```python
from build123d import *
from OCP.BRepFilletAPI import BRepFilletAPI_MakeChamfer

# Parameters (mm, degrees)
SKETCH_1_W          = 23
SKETCH_1_H          = 40
SKETCH_1_R          = 9.5
EXTRUDE_1_DEPTH     = 1.5
FILLET_1_R          = 2
SKETCH_3_R          = 1.15
CUT_EXTRUDE_1_DEPTH = 24.119256043
SKETCH_4_R          = 0.65
EXTRUDE_2_DEPTH     = 2
CHAMFER_1_SIZE      = 2
CHAMFER_1_SIZE_2    = 0.1


with BuildPart() as part:
    # 草图1 → 凸台-拉伸1 (new body)
    with BuildSketch(Plane.XY):
        Rectangle(SKETCH_1_W, SKETCH_1_H)
        with Locations((0, -4.5)):
            Circle(SKETCH_1_R, mode=Mode.SUBTRACT)
    extrude(amount=EXTRUDE_1_DEPTH)

    # 圆角1
    fillet_1_edges = [part.edges().sort_by_distance(p)[0] for p in [
        (11.5, -20, 0.75),
        (-11.5, -20, 0.75),
        (-11.5, 20, 0.75),
        (11.5, 20, 0.75),
    ]]
    fillet(fillet_1_edges, radius=FILLET_1_R)

    # 草图3 → 切除-拉伸1 (cut, through all)
    with BuildSketch(Plane.XY.offset(1.5)):
        with Locations((-8, 18)):
            Circle(SKETCH_3_R)
        with Locations((8, 18)):
            Circle(SKETCH_3_R)
        with Locations((-9, -17)):
            Circle(SKETCH_3_R)
        with Locations((9, -17)):
            Circle(SKETCH_3_R)
    extrude(amount=-CUT_EXTRUDE_1_DEPTH, mode=Mode.SUBTRACT)

    # 草图4 → 凸台-拉伸2 (add)
    with BuildSketch(Plane.XY.offset(1.5)):
        with Locations(Location((-8, -12, 0), (0, 0, 180))):
            Circle(SKETCH_4_R)
        with Locations(Location((8, -12, 0), (0, 0, 180))):
            Circle(SKETCH_4_R)
    extrude(amount=EXTRUDE_2_DEPTH)

    # 倒角1
    chamfer_1_edges_1 = [part.edges().sort_by_distance(p)[0] for p in [
        (-7.35, -12, 3.5),
    ]]
    chamfer_1_side_1 = [part.faces().sort_by_distance(p)[0] for p in [
        (-7.35, -12, 3.498),
    ]]
    chamfer_1_edges_2 = [part.edges().sort_by_distance(p)[0] for p in [
        (8.65, -12, 3.5),
    ]]
    chamfer_1_side_2 = [part.faces().sort_by_distance(p)[0] for p in [
        (8.65, -12, 3.498),
    ]]
    chamfer_1 = BRepFilletAPI_MakeChamfer(part.part.solid().wrapped)
    for e in chamfer_1_edges_1:
        chamfer_1.Add(CHAMFER_1_SIZE - 0.0001, CHAMFER_1_SIZE_2 - 0.0001, e.wrapped, chamfer_1_side_1[0].wrapped)
    for e in chamfer_1_edges_2:
        chamfer_1.Add(CHAMFER_1_SIZE - 0.0001, CHAMFER_1_SIZE_2 - 0.0001, e.wrapped, chamfer_1_side_2[0].wrapped)
    add(Compound.cast(chamfer_1.Shape()), mode=Mode.REPLACE)  # a hair under: the kernel refuses the full size


solid = part.part
```
For this review, take the finished solid that the model builds, in its own axes (mm). Round coordinates to 2 decimals unless told otherwise and drop trailing zeros. Write each loop counter-clockwise with the first axis right and the second up, starting at its lowest first coordinate (ties: lowest second). Pieces come first, ordered by that corner, then holes.
1) Take a section at B-B on z = 0.45. Give the boundary of the cut face in (x, y), then the cut area to 3 significant figures.
Answer below:
outline: (-11.5, -18) arc R2 ccw to (-9.5, -20) - (9.5, -20) arc R2 ccw to (11.5, -18) - (11.5, 18) arc R2 ccw to (9.5, 20) - (-9.5, 20) arc R2 ccw to (-11.5, 18) - close; hole circle Ø2.3 at (-9, -17); hole circle Ø19 at (0, -4.5); hole circle Ø2.3 at (-8, 18); hole circle Ø2.3 at (8, 18); hole circle Ø2.3 at (9, -17)
area: 616 mm2
2) Take a section at D-D on x = -6. Give the boundary of the cut face in (y, z), then the cut area to 3 significant figures.
Answer below:
outline: (-20, 0) - (-11.87, 0) - (-11.87, 1.5) - (-20, 1.5) - close; (2.87, 0) - (20, 0) - (20, 1.5) - (2.87, 1.5) - close
area: 37.9 mm2
3) Take a section at C-C on y = -4.5. Give the boundary of the cut face in (x, z).
Answer below:
outline: (-11.5, 0) - (-9.5, 0) - (-9.5, 1.5) - (-11.5, 1.5) - close; (9.5, 0) - (11.5, 0) - (11.5, 1.5) - (9.5, 1.5) - close
4) Mouldability with a two-part tool opening along Y and no side actions: class faces 1 (the face through (10.9, 19.43, 0.76)), 2 (the face through (-10.93, -19.4, 0.76)), 3 (the face through (-7.903, -16.655, 0.76)), 4 (the face through (-7.47, 16.98, 0.76)) as +Y half, -Y half, draft (parallel to the pull), parting line (faces both ways), or undercut.
Answer below:
face 1: +Y half
face 2: -Y half
face 3: undercut
face 4: undercut
5) Insertion check: pin 1 Ø10 at (x, y) = (0, 8.5) entering from +Z. The pin has a flat end and moves straight along its axis. Give the tip position at first contact, or say it passes through.
Answer below:
pin 1: stops at z = 1.5
6) For line 1 along Y through (x, z) = (0, 0.75); line 2 along Y through (x, z) = (-7.75, 1.35); line 3 along Y through (x, z) = (8, 0.4), list the stretches that pass through material, from the lowest coordinate up.
Answer below:
line 1: y = -20 to -14, 5 to 20
line 2: y = -20 to -9.99, 0.99 to 16.88, 19.12 to 20
line 3: y = -20 to -17.57, -16.43 to -9.62, 0.62 to 16.85, 19.15 to 20
7) Take a section at A-A on y = -17. Give the boundary of the cut face in (x, z), then the cut area to 3 significant figures.
Answer below:
outline: (-11.5, 0) - (-10.15, 0) - (-10.15, 1.5) - (-11.5, 1.5) - close; (-7.85, 0) - (7.85, 0) - (7.85, 1.5) - (-7.85, 1.5) - close; (10.15, 0) - (11.5, 0) - (11.5, 1.5) - (10.15, 1.5) - close
area: 27.6 mm2
